Design review of the part built by this model. Coordinates are the model's own, in mm. A direction names the side the tool comes from. Coordinates: 2 decimals unless noted, no trailing zeros. Loops run counter-clockwise (first coordinate to the right, second up) from the corner with the lowest first, then second, coordinate; pieces in that order, holes last. Notation, with made-up numbers: (7, -6.5) - (34, -6.5) arc R17 cw to (34, -0.5) - close; hole circle Ø11 at (46, 56.25). An arc over 180 degrees is marked (long way). One line per question, with ' | ' between items.
Autodesk Inventor part; units mm, degrees
ref_plane "YZ Plane" through (0, 0, 0) normal (1, 0, 0) x (0, 1, 0)
ref_plane "XZ Plane" through (0, 0, 0) normal (0, 1, 0) x (-1, 0, 0)
ref_plane "XY Plane" through (0, 0, 0) normal (0, 0, 1) x (1, 0, 0)
sketch "Sketch1" plane through (0, 0, 0) normal (0, 1, 0) x (-1, 0, 0)
  line L0 (0, 0) -> (12.7, 0)
  line L1 (12.7, 0) -> (12.7, 33.02)
  line L2 (12.7, 33.02) -> (0, 33.02)
  line L3 (0, 33.02) -> (0, 0)
  dimension "d0" = 12.7
  dimension "d1" = 33.02
extrude "Extrusion1" add sketch "Sketch1" along normal blind 2.286
sketch "Sketch2" plane through (0, 2.286, 0) normal (0, 1, 0) x (1, 0, 0)
  point P0 (0, 0)
sketch "Sketch3" plane through (0, 2.286, 0) normal (0, 1, 0) x (1, 0, 0)
  circle A0 centre (-6.35, -6.35) radius 1.778
  point P0 (0, 0)
  dimension "d4" = 3.556
hole "Hole1" at (-6.35, 2.286, 6.35) direction (0, -1, 0) diameter 3.175 end through all
sketch "Sketch4" plane through (0, 2.286, 0) normal (0, 1, 0) x (1, 0, 0)
  point P0 (0, 0)
sketch "Sketch6" plane through (0, 2.286, 0) normal (0, 1, 0) x (1, 0, 0)
  line L0 (-6.35, -15.875) -> (-6.35, -28.575) construction
  line L1 (-7.9375, -15.875) -> (-7.9375, -28.575)
  line L2 (-4.7625, -28.575) -> (-4.7625, -15.875)
  arc A0 (-4.7625, -15.875) -> (-7.9375, -15.875) centre (-6.35, -15.875) ccw
  arc A1 (-7.9375, -28.575) -> (-4.7625, -28.575) centre (-6.35, -28.575) ccw
  point P0 (0, 0)
  point P1 (-6.35, -12.7)
  point P2 (-6.35, -22.225)
  dimension "d15" = 3.175
extrude "Extrusion3" cut sketch "Sketch6" against normal blind 2.286
sketch "Sketch7" plane through (0, 2.286, 0) normal (0, 1, 0) x (1, 0, 0)
  circle A0 centre (-6.35, -6.35) radius 1.5875
  circle A1 centre (-6.35, -6.35) radius 3.175
  point P0 (0, 0)
  dimension "d18" = 6.35
properties part number "WireHangerBase"
Q1. Tool access review of faces 1 (the cylindrical face through (-6.315, 1.159, 14.288)), 2 (the flat face through (0, 1, 17)): name each direction out of +Z, -Z, +X, -X, +Y, -Y from which nothing blocks a thin tool from reaching the whole face with its end or side.
Returned:
face 1: +Y, -Y | face 2: +Z, -Z, +X, +Y, -Y
Q2. Draft analysis for pull direction X (two halves, no side actions). For faces 3 (the flat face through (-7.938, 1, 22)), 4 (the flat face through (-12.7, 1, 16)), 5 (the flat face through (-4.762, 1, 22)), 6 (the flat face through (-6, 1, 33.02)), state which applies: +X half, -X half, draft (parallel to the pull), parting line (faces both ways), or undercut.
Returned:
face 3: undercut | face 4: -X half | face 5: undercut | face 6: draft
Q3. To check wall thickness, follow line 1 along Z through (x, y) = (-6.35, 1); line 2 along X through (y, z) = (1.6, 23). State the ranges of each line that lie inside material, in increasing order.
Returned:
line 1: z = 0 to 4.76, 7.94 to 14.29, 30.16 to 33.02 | line 2: x = -12.7 to -7.94, -4.76 to 0
Q4. Take a section at B-B (z = 26). Give the boundary of the cut face in (x, y).
Returned:
outline: (-12.7, 0) - (-7.94, 0) - (-7.94, 2.29) - (-12.7, 2.29) - close; (-4.76, 0) - (0, 0) - (0, 2.29) - (-4.76, 2.29) - close
Q5. Take a section at A-A (x = -6.35). Give the boundary of the cut face in (y, z), plus the area to 3 significant figures.
Returned:
outline: (0, 0) - (2.29, 0) - (2.29, 4.76) - (0, 4.76) - close; (0, 7.94) - (2.29, 7.94) - (2.29, 14.29) - (0, 14.29) - close; (0, 30.16) - (2.29, 30.16) - (2.29, 33.02) - (0, 33.02) - close | area: 31.9 mm²
Q6. Take a section at C-C (y = 0.75). State how many separate pieces and enclosed holes the cut face has, plus the area to 3 significant figures.
Returned:
separate pieces: 1 | enclosed holes: 2 | area: 363 mm²
